from build123d import *

# Parameters (mm, degrees)
EXTRU_MINCE3_DEPTH = 15
BOSS_EXTRU_2_DEPTH = 5


with BuildPart() as part:
    # Esquisse1 → Extru.-Mince3 (new body)
    with BuildSketch(Plane.XY):
        with BuildLine():
            Line((5, -5), (95, -5))
            ThreePointArc((95, -5), (102.071067812, -2.071067812), (105, 5))
            Line((105, 5), (105, 45))
            ThreePointArc((105, 45), (102.071067812, 52.071067812), (95, 55))
            Line((95, 55), (5, 55))
            ThreePointArc((5, 55), (-2.071067812, 52.071067812), (-5, 45))
            Line((-5, 45), (-5, 5))
            ThreePointArc((-5, 5), (-2.071067812, -2.071067812), (5, -5))
        make_face()
        with BuildLine():
            Line((5, 0), (95, 0))
            ThreePointArc((95, 0), (98.535533906, 1.464466094), (100, 5))
            Line((100, 5), (100, 45))
            ThreePointArc((100, 45), (98.535533906, 48.535533906), (95, 50))
            Line((95, 50), (5, 50))
            ThreePointArc((5, 50), (1.464466094, 48.535533906), (0, 45))
            Line((0, 45), (0, 5))
            ThreePointArc((0, 5), (1.464466094, 1.464466094), (5, 0))
        make_face(mode=Mode.SUBTRACT)
    extrude(amount=EXTRU_MINCE3_DEPTH)

    # Esquisse2 → Boss.-Extru.2 (add)
    with BuildSketch(Plane.XY):
        with BuildLine():
            Line((5, 50), (95, 50))
            ThreePointArc((95, 50), (98.535533906, 48.535533906), (100, 45))
            Line((100, 45), (100, 5))
            ThreePointArc((100, 5), (98.535533906, 1.464466094), (95, 0))
            Line((95, 0), (5, 0))
            ThreePointArc((5, 0), (1.464466094, 1.464466094), (0, 5))
            Line((0, 5), (0, 45))
            ThreePointArc((0, 45), (1.464466094, 48.535533906), (5, 50))
        make_face()
    extrude(amount=BOSS_EXTRU_2_DEPTH)


solid = part.part
Read the model definition and answer for the solid it produces. Units are mm, in the model's axes. A direction names the side the tool comes from. Give positions to 0.01 mm unless a question says otherwise; leave off trailing zeros. Write each loop counter-clockwise with the first axis right and the second up, starting at its lowest first coordinate (ties: lowest second). Pieces come first, ordered by that corner, then holes. Notation, with made-up numbers: M 89.25,3 L 120.25,3 A30 cw 120.25,41 Z; hole C -8,75 d2. An arc over 180 degrees is marked long. One line per item, written item: value. Start each with the question number.
(1) Find section C-C (z = 6.5). Determine the outline of the cut face in (x, y).
(2) Flat-ended cylindrical pins translate along their axes: pin 1 Ø2 at (y, z) = (47, 5) entering from -X; pin 2 Ø15 at (x, y) = (52.5, 27.5) entering from +Z. Find the tip coordinate at first contact, or state that the pin passes through.
(3) Find the intervals of material crossed by line 1 (Y direction, x = 45, z = 12); line 2 (X direction, y = 31, z = 13.25); line 3 (Z direction, x = 87.5, y = 29), in increasing order.
(4) Find section B-B (x = 16). Determine the outline of the cut face in (y, z).
(5) Find section A-A (y = 20.5). Determine the outline of the cut face in (x, z).
(6) Determine the mould class of faces 3 (the flat face through (0, 25, 10)), 4 (the cylindrical face through (-2.15, -1.99, 7.4)), 5 (the flat face through (46, -2, 15)) for opening direction X: pulls with the +X half, pulls with the -X half, needs draft (parallel to the pull), parting line crosses it, or undercut.
(7) A tool of negligible diameter and unlimited length cuts with its end or side. For faces 1 (the flat face through (51, 55, 7)), 2 (the cylindrical face through (99, 48, 10)), from which of +Z, -Z, +X, -X, +Y, -Y can it reach the whole face along a straight path? Write none if from no direction.
Results below:
1. outline: M -5,5 A10 ccw 5,-5 L 95,-5 A10 ccw 105,5 L 105,45 A10 ccw 95,55 L 5,55 A10 ccw -5,45 Z; hole M 0,5 A5 ccw 5,0 L 95,0 A5 ccw 100,5 L 100,45 A5 ccw 95,50 L 5,50 A5 ccw 0,45 Z
2. pin 1: stops at x = -4.95
2. pin 2: stops at z = 5
3. line 1: y = -5 to 0, 50 to 55
3. line 2: x = -5 to 0, 100 to 105
3. line 3: z = 0 to 5
4. outline: M -5,0 L 55,0 L 55,15 L 50,15 L 50,5 L 0,5 L 0,15 L -5,15 Z
5. outline: M -5,0 L 105,0 L 105,15 L 100,15 L 100,5 L 0,5 L 0,15 L -5,15 Z
6. face 3: undercut
6. face 4: pulls with the -X half
6. face 5: needs draft
7. face 1: +Z, -Z, +X, -X, +Y
7. face 2: +Z
